Part model, mm, in its own coordinate system. Face numbers are marked on the shaded views. A direction names the side the tool comes from. Give positions to 0.01 mm unless a question says otherwise; leave off trailing zeros. Order: outer loops, then holes, each group sorted by start corner. A loop starts at its lowest first (then second) coordinate and runs counter-clockwise, first axis right, second up. Notation, with made-up numbers: (-29.5, 58.5) - (-25.5, 58.5) arc R29 ccw to (-25.5, 92.5) - close; hole circle Ø5 at (-6, 28.5). An arc over 180 degrees is marked (long way). One line per item, written item: value.
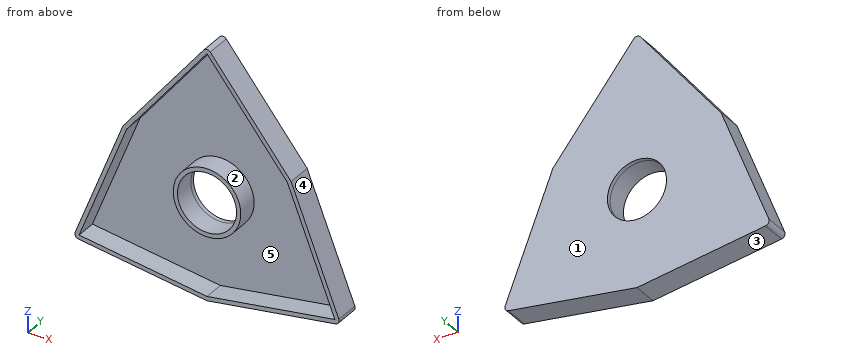
```python
from build123d import *

# Parameters (mm, degrees)
F0_R     = 8
F0_R_2   = 7
F1_DEPTH = 1
F2_DEPTH = 5


with BuildPart() as f1:
    # F0 (on Front) → F1 (new body)
    with BuildSketch(Plane.XZ):
        with BuildLine():
            Line((-19.928076, 11.50548), (-31.240951, -17.132598))
            ThreePointArc((-31.240951, -17.132598), (-31.176915, -18), (-30.457741, -18.489158))
            Line((-30.457741, -18.489158), (0, -23.01096))
            Line((0, -23.01096), (30.457741, -18.489158))
            ThreePointArc((30.457741, -18.489158), (31.176915, -18), (31.240951, -17.132598))
            Line((31.240951, -17.132598), (19.928076, 11.50548))
            Line((19.928076, 11.50548), (0.78321, 35.621757))
            ThreePointArc((0.78321, 35.621757), (0, 36), (-0.78321, 35.621757))
            Line((-0.78321, 35.621757), (-19.928076, 11.50548))
        make_face()
        Polygon((0, -22), (-30.310889, -17.5), (-19.052559, 11), (0, 35), (19.052559, 11), (30.310889, -17.5), align=None, mode=Mode.SUBTRACT)
        Polygon((-19.052559, 11), (-30.310889, -17.5), (0, -22), (30.310889, -17.5), (19.052559, 11), (0, 35), align=None)
        Circle(F0_R, mode=Mode.SUBTRACT)
        Circle(F0_R)
        Circle(F0_R_2, mode=Mode.SUBTRACT)
    extrude(amount=-F1_DEPTH)

    # F0 (on Front) → F2 (join)
    with BuildSketch(Plane.XZ):
        with BuildLine():
            Line((-19.928076, 11.50548), (-31.240951, -17.132598))
            ThreePointArc((-31.240951, -17.132598), (-31.176915, -18), (-30.457741, -18.489158))
            Line((-30.457741, -18.489158), (0, -23.01096))
            Line((0, -23.01096), (30.457741, -18.489158))
            ThreePointArc((30.457741, -18.489158), (31.176915, -18), (31.240951, -17.132598))
            Line((31.240951, -17.132598), (19.928076, 11.50548))
            Line((19.928076, 11.50548), (0.78321, 35.621757))
            ThreePointArc((0.78321, 35.621757), (0, 36), (-0.78321, 35.621757))
            Line((-0.78321, 35.621757), (-19.928076, 11.50548))
        make_face()
        Polygon((0, -22), (-30.310889, -17.5), (-19.052559, 11), (0, 35), (19.052559, 11), (30.310889, -17.5), align=None, mode=Mode.SUBTRACT)
        Circle(F0_R)
        Circle(F0_R_2, mode=Mode.SUBTRACT)
    extrude(amount=F2_DEPTH)


solid = f1.part
```
1) Cut at B-B, the plane z = 4.5. Give the cut face in (x, y).
Outcome:
outline: (-22.7, -5) - (-21.62, -5) - (-21.62, 0) - (-6.61, 0) - (-6.61, -5) - (-5.36, -5) - (-5.36, 1) - (-22.7, 1) - close; (5.36, -5) - (6.61, -5) - (6.61, 0) - (21.62, 0) - (21.62, -5) - (22.7, -5) - (22.7, 1) - (5.36, 1) - close
2) Mould opens along X. For the marked faces 3, 4 and 5 say: released by +X, released by -X, zero draft, split by the parting line, or undercut.
Outcome:
face 3: released by -X
face 4: released by +X
face 5: undercut
3) Which spindle directions (+Z, -Z, +X, -X, +Y, -Y) get a long thin tool onto all of the face, cutting with end or side? Do the marked faces 1 and 2. Say none if no direction does.
Outcome:
face 1: +Z, -Z, +X, -X, +Y
face 2: -Y
4) Pin check, flat tips, straight feed: pin 1 (2 mm diameter, centred on y = -3, z = 21, fed in from +X); pin 2 (2 mm diameter, centred on y = -2.5, z = -11.5, fed in from -X). Stop position of each tip, or through.
Outcome:
pin 1: stops at x = 13.18
pin 2: stops at x = -29.41
5) Cut at C-C, the plane z = 28.5. Give the cut face in (x, y).
Outcome:
outline: (-6.44, -5) - (-5.16, -5) - (-5.16, 0) - (5.16, 0) - (5.16, -5) - (6.44, -5) - (6.44, 1) - (-6.44, 1) - close
6) Drill centre lines: line 1 along Z through (x, y) = (-2, -2.5); line 2 along X through (y, z) = (-2.75, 6); line 3 along X through (y, z) = (-4.1, 1). Where is each one in solid material? Low to high. Write a range as from..to.
Outcome:
line 1: z = -22.71..-21.7, -7.75..-6.71, 6.71..7.75, 32.48..34.09
line 2: x = -22.1..-21.03, -5.29..-3.61, 3.61..5.29, 21.03..22.1
line 3: x = -24.08..-23, -7.94..-6.93, 6.93..7.94, 23..24.08
7) Cut at A-A, the plane y = -1.55. Give the cut face in (x, z), then the cut area to 3 significant figures.
Outcome:
outline: (-31.24, -17.13) arc R1 ccw to (-30.46, -18.49) - (0, -23.01) - (30.46, -18.49) arc R1 ccw to (31.24, -17.13) - (19.93, 11.51) - (0.78, 35.62) arc R1 ccw to (-0.78, 35.62) - (-19.93, 11.51) - close; circle Ø16 at (0, 0); hole (-30.31, -17.5) - (0, -22) - (30.31, -17.5) - (19.05, 11) - (0, 35) - (-19.05, 11) - close; hole circle Ø14 at (0, 0)
area: 234 mm^2
8) Cut at D-D, the plane x = 27. Give the cut face in (y, z), then the cut area to 3 significant figures.
Outcome:
outline: (-5, -19) - (1, -19) - (1, -6.4) - (-5, -6.4) - (-5, -9.12) - (0, -9.12) - (0, -17.99) - (-5, -17.99) - close
area: 31.3 mm^2
